Geometry: final body of the model. Coordinates: model frame, mm. Round coordinates to 2 decimals unless told otherwise and drop trailing zeros. Order: outer loops, then holes, each group sorted by start corner. A loop starts at its lowest first (then second) coordinate and runs counter-clockwise, first axis right, second up. Notation, with made-up numbers: (-33.75, -24) - (19.25, -24) arc R7 ccw to (19.25, -12) - close; hole circle Ø9 at (-34, 73.25). An arc over 180 degrees is marked (long way). Put each result on its own line as item: value. Start each with the question number.
(1) Section B-B (z = 0). Output: boundary loops of the cut face in (x, y), and give its area (3 significant figures).
(2) Pin query (flat end, axial travel): P1, Ø3, axis at x = 24, z = -1.5, coming from the +Y side. Return the tip coordinate at first contact, or that it passes through.
(3) Section A-A (x = 0). Output: boundary loops of the cut face in (y, z), and give its area (3 significant figures).
(4) Material intervals for L1, parallel to Z at x = 0, y = -1.05; L2, parallel to Z at x = 31, y = -1.4; L3, parallel to X at y = -2.05, z = 14, sorted ascending. Write a range as [from, to].
(5) Section C-C (x = -31). Output: boundary loops of the cut face in (y, z).
(6) Section D-D (z = -23). Output: boundary loops of the cut face in (x, y).
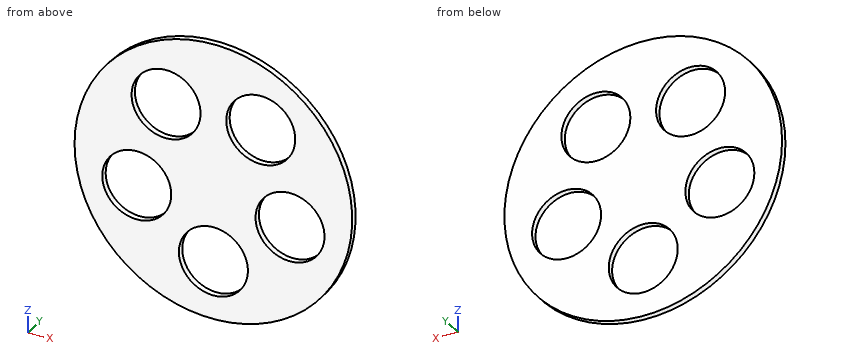
Autodesk Inventor part; units mm, degrees
ref_plane "YZ Plane" through (0, 0, 0) normal (1, 0, 0) x (0, 1, 0)
ref_plane "XZ Plane" through (0, 0, 0) normal (0, 1, 0) x (-1, 0, 0)
ref_plane "XY Plane" through (0, 0, 0) normal (0, 0, 1) x (1, 0, 0)
sketch "Sketch1" plane through (0, 0, 0) normal (0, 1, 0) x (-1, 0, 0)
  circle A0 centre (0, 0) radius 57.4978
  circle A1 centre (0, 0) radius 33.3678 construction
  circle A2 centre (0, -33.3678) radius 14.2875
  circle A3 centre (31.7347, -10.3112) radius 14.2875
  circle A4 centre (19.6131, 26.9951) radius 14.2875
  circle A5 centre (-19.6131, 26.9951) radius 14.2875
  circle A6 centre (-31.7347, -10.3112) radius 14.2875
  dimension "wheelFilterDiameter" = 66.7357
  dimension "wheelOuterDiameter" = 114.9957
  dimension "filterThreadDiameter" = 28.575
  dimension "d5" = 360
extrude "Extrusion1" add sketch "Sketch1" against normal blind 2.54
thread "Thread1"
equation "\"wheelFilterDiameter\" = 0.318471 * wheelFilterCircumference"
equation "\"wheelOuterDiameter\" = filterDiameter + wheelFilterDiameter + 2 * distanceFromFilterToEdge"
equation "\"distanceBetweenFilters\" = 12.7"
equation "\"distanceFromFilterToEdge\" = 9.525"
equation "\"filterDiameter\" = 29.21"
properties part number "filterHolder"
Checks:
1. outline: (-57.5, -2.54) - (-41.62, -2.54) - (-41.62, 0) - (-57.5, 0) - close; (-21.84, -2.54) - (21.84, -2.54) - (21.84, 0) - (-21.84, 0) - close; (41.62, -2.54) - (57.5, -2.54) - (57.5, 0) - (41.62, 0) - close
1. area: 192 mm²
2. P1: passes through
3. outline: (-2.54, -57.5) - (0, -57.5) - (0, -47.66) - (-2.54, -47.66) - close; (-2.54, -19.08) - (0, -19.08) - (0, 57.5) - (-2.54, 57.5) - close
3. area: 220 mm²
4. L1: z = [-57.5, -47.66], [-19.08, 57.5]
4. L2: z = [-48.43, -24.58], [3.96, 18.37], [35.62, 48.43]
4. L3: x = [-55.77, -25.55], [-13.68, 13.68], [25.55, 55.77]
5. outline: (-2.54, -48.43) - (0, -48.43) - (0, -24.58) - (-2.54, -24.58) - close; (-2.54, 3.96) - (0, 3.96) - (0, 18.37) - (-2.54, 18.37) - close; (-2.54, 35.62) - (0, 35.62) - (0, 48.43) - (-2.54, 48.43) - close
6. outline: (-52.7, -2.54) - (-38.3, -2.54) - (-38.3, 0) - (-52.7, 0) - close; (-25.17, -2.54) - (-9.83, -2.54) - (-9.83, 0) - (-25.17, 0) - close; (9.83, -2.54) - (25.17, -2.54) - (25.17, 0) - (9.83, 0) - close; (38.3, -2.54) - (52.7, -2.54) - (52.7, 0) - (38.3, 0) - close
